Check sheet for the modelled part. Datum: model origin and axes. Units: mm. Round coordinates to 2 decimals unless told otherwise and drop trailing zeros. Loops run counter-clockwise (first coordinate to the right, second up) from the corner with the lowest first, then second, coordinate; pieces in that order, holes last. Notation, with made-up numbers: (18.25, 1.5) -> (58.25, 1.5) arc R20 cw to (58.25, 32.5) -> close; hole circle Ø8 at (15, 35.25). An arc over 180 degrees is marked (long way). Return JSON: item names as keys, results as strings.
from build123d import *

# Parameters (mm, degrees)
F1_DEPTH = 15


with BuildPart() as f1:
    # F0 (on Right) → F1 (new body)
    with BuildSketch(Plane.YZ):
        with BuildLine():
            ThreePointArc((-100, 82.879485), (-135.930106, 67.650557), (-149.973133, 31.240583))
            Line((-149.973133, 31.240583), (-227.556466, -482.939178))
            Line((-227.556466, -482.939178), (-212.724353, -485.177159))
            Line((-212.724353, -485.177159), (-144.362209, -32.110378))
            Line((-144.362209, -32.110378), (144.362209, -32.110378))
            Line((144.362209, -32.110378), (212.724353, -485.177159))
            Line((212.724353, -485.177159), (227.556466, -482.939178))
            Line((227.556466, -482.939178), (149.973133, 31.240583))
            ThreePointArc((149.973133, 31.240583), (135.930106, 67.650557), (100, 82.879485))
            Line((100, 82.879485), (0, 82.879485))
            Line((0, 82.879485), (-100, 82.879485))
        make_face()
        with BuildLine():
            Line((-142.098895, -17.110378), (-134.91779, 30.482052))
            ThreePointArc((-134.91779, 30.482052), (-125.582317, 56.765564), (-100, 67.879481))
            Line((-100, 67.879481), (0, 67.879481))
            Line((0, 67.879481), (100, 67.879481))
            ThreePointArc((100, 67.879481), (125.582317, 56.765564), (134.91779, 30.482052))
            Line((134.91779, 30.482052), (142.098895, -17.110378))
            Line((142.098895, -17.110378), (-142.098895, -17.110378))
        make_face(mode=Mode.SUBTRACT)
    extrude(amount=F1_DEPTH)


solid = f1.part
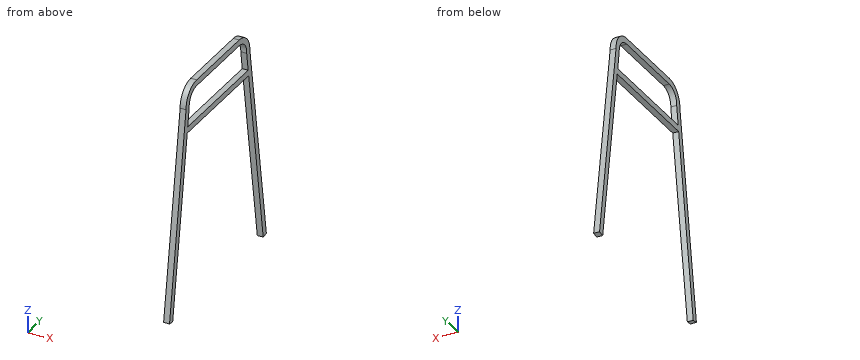
Q1. Section check A-A (y = 78). Record the boundary of the cut face in (x, z), then the cut area to 3 significant figures.
Results list:
{"outline": "(0, -32.11) -> (15, -32.11) -> (15, -17.11) -> (0, -17.11) -> close; (0, 67.88) -> (15, 67.88) -> (15, 82.88) -> (0, 82.88) -> close", "area": "450 mm^2"}
Q2. Section check C-C (z = -4.5). Record the boundary of the cut face in (x, y).
Results list:
{"outline": "(0, -155.37) -> (15, -155.37) -> (15, -140.2) -> (0, -140.2) -> close; (0, 140.2) -> (15, 140.2) -> (15, 155.37) -> (0, 155.37) -> close"}
Q3. Material ranges on line 1 (Z direction, x = 6.25, y = 8.5); line 2 (Y direction, x = 11, z = -414); line 3 (Z direction, x = 3, y = -111.5), recorded low to high.
Results list:
{"line 1": "-32.11 to -17.11, 67.88 to 82.88", "line 2": "-217.15 to -201.98, 201.98 to 217.15", "line 3": "-32.11 to -17.11, 65.94 to 81.54"}
Q4. Section check D-D (y = 166.5). Record the boundary of the cut face in (x, z).
Results list:
{"outline": "(0, -178.83) -> (15, -178.83) -> (15, -78.29) -> (0, -78.29) -> close"}
Q5. Go/stop test with flat-tipped pins: pin 1 (4.5 mm diameter, centred on x = 9, y = -33, fed in from -Z); pin 2 (2 mm diameter, centred on x = 2.5, z = -346.5, fed in from -Y); pin 3 (2 mm diameter, centred on x = 10, z = -8, fed in from +Y). Record where each tip stops, or that it passes through.
Results list:
{"pin 1": "z = -32.11", "pin 2": "y = -207.12", "pin 3": "y = 156.04"}
Q6. Section check B-B (x = 12). Record the boundary of the cut face in (y, z), then the cut area to 3 significant figures.
Results list:
{"outline": "(-227.56, -482.94) -> (-212.72, -485.18) -> (-144.36, -32.11) -> (144.36, -32.11) -> (212.72, -485.18) -> (227.56, -482.94) -> (149.97, 31.24) arc R50 ccw to (100, 82.88) -> (-100, 82.88) arc R50 ccw to (-149.97, 31.24) -> close; hole (-142.1, -17.11) -> (142.1, -17.11) -> (134.92, 30.48) arc R35 ccw to (100, 67.88) -> (-100, 67.88) arc R35 ccw to (-134.92, 30.48) -> close", "area": "25,000 mm^2"}
